The listing builds one solid part. Answer for the finished solid, in the listing's coordinates (mm). Face numbers are marked on the shaded views. A direction names the side the tool comes from. Round coordinates to 2 decimals unless told otherwise and drop trailing zeros. Order: outer loops, then holes, each group sorted by start corner. A loop starts at its lowest first (then second) coordinate and runs counter-clockwise, first axis right, second up. Notation, with made-up numbers: (60, -18) - (81, -18) arc R26 cw to (81, 0) - close; hole circle Ø11 at (-26.75, 39). An arc over 180 degrees is marked (long way). One line per item, written item: value. Start each with the question number.
1. For a pull along Z with two mould halves and no side action, classify the marked faces 3, 4 and 5 as released by +Z, released by -Z, zero draft, split by the parting line, or undercut.
2. Section D-D, the plane y = 2.65 is taken. Give the vertices of the cut face in (x, z).
3. Section C-C, the plane y = 0.4 is taken. Give the vertices of the cut face in (x, z).
4. A tool of negligible diameter and unlimited length cuts with its end or side. For the marked faces 1 and 2, from which of +Z, -Z, +X, -X, +Y, -Y can it reach the whole face along a straight path? Write none if from no direction.
5. Flat-ended cylindrical pins translate along their axes: P1, Ø2, axis at x = -3, y = 3.5, coming from the -Z side; P2, Ø4, axis at x = 0, z = 0, coming from the +Y side; P3, Ø2, axis at x = -4.5, y = 3, coming from the +Z side. Find the tip coordinate at first contact, or state that the pin passes through.
6. Straight lines are drawn through the part: line 1 (X direction, y = 0.8, z = 0); line 2 (X direction, y = 1.75, z = 0); line 3 (X direction, y = 3.5, z = -1.5). For each, find the intervals that lie inside material, in ascending order.
7. Section A-A, the plane x = -1.25 is taken. Give the vertices of the cut face in (y, z), then the cut area to 3 significant figures.
8. Section B-B, the plane z = 0 is taken. Give the vertices of the cut face in (x, y), then the cut area to 3 significant figures.
from build123d import *

# Parameters (mm, degrees)
SKETCH1_R           = 5
SKETCH1_R_2         = 2.5
BOSS_EXTRUDE1_DEPTH = 3.2
SKETCH2_R           = 5.8
SKETCH2_R_2         = 2.5
BOSS_EXTRUDE2_DEPTH = 0.8
SKETCH3_R           = 4.35508582
SKETCH3_R_2         = 3.692114727
CUT_EXTRUDE1_DEPTH  = 1
SKETCH4_R           = 4.43730614
SKETCH4_R_2         = 3.629860823
CUT_EXTRUDE2_DEPTH  = 1


with BuildPart() as part:
    # Sketch1 → Boss-Extrude1 (new body)
    with BuildSketch(Plane(origin=(0, 0, 0), x_dir=(1, 0, 0), z_dir=(0, 1, 0))):
        with Locations(Location((0, 0, 0), (0, 0, 270))):
            Circle(SKETCH1_R)
        with Locations(Location((0, 0, 0), (0, 0, 270))):
            Circle(SKETCH1_R_2, mode=Mode.SUBTRACT)
    extrude(amount=BOSS_EXTRUDE1_DEPTH)

    # Sketch2 → Boss-Extrude2 (add)
    with BuildSketch(Plane(origin=(0, 3.2, 0), x_dir=(1, 0, 0), z_dir=(0, 1, 0))):
        with Locations(Location((0, 0, 0), (0, 0, 270))):
            Circle(SKETCH2_R)
        with Locations(Location((0, 0, 0), (0, 0, 270))):
            Circle(SKETCH2_R_2, mode=Mode.SUBTRACT)
    extrude(amount=BOSS_EXTRUDE2_DEPTH)

    # Sketch3 → Cut-Extrude1 (cut)
    with BuildSketch(Plane.XZ):
        with Locations(Location((0, 0, 0), (0, 0, 270))):
            Circle(SKETCH3_R)
        with Locations(Location((0, 0, 0), (0, 0, 270))):
            Circle(SKETCH3_R_2, mode=Mode.SUBTRACT)
    extrude(amount=-CUT_EXTRUDE1_DEPTH, mode=Mode.SUBTRACT)

    # Sketch4 → Cut-Extrude2 (cut)
    with BuildSketch(Plane(origin=(0, 4, 0), x_dir=(1, 0, 0), z_dir=(0, 1, 0))):
        with Locations(Location((0, 0, 0), (0, 0, 270))):
            Circle(SKETCH4_R)
        with Locations(Location((0, 0, 0), (0, 0, 270))):
            Circle(SKETCH4_R_2, mode=Mode.SUBTRACT)
    extrude(amount=-CUT_EXTRUDE2_DEPTH, mode=Mode.SUBTRACT)


solid = part.part
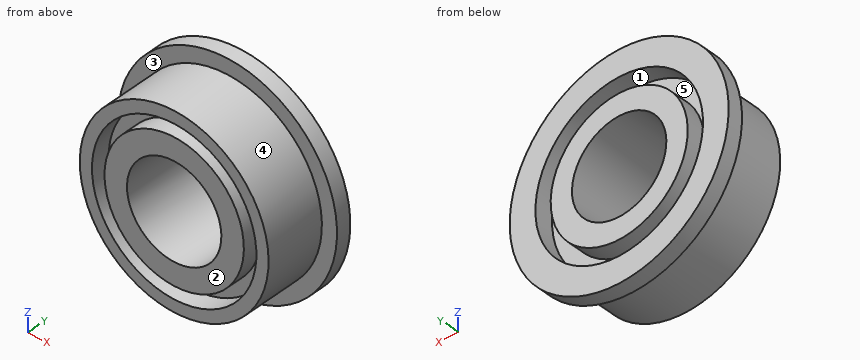
Answer list:
1. face 3: zero draft
1. face 4: split by the parting line
1. face 5: undercut
2. outline: circle Ø10 at (0, 0); hole circle Ø5 at (0, 0)
3. outline: circle Ø10 at (0, 0); circle Ø7.38 at (0, 0); hole circle Ø8.71 at (0, 0); hole circle Ø5 at (0, 0)
4. face 1: +Y
4. face 2: +Z, -Z, +X, -X, -Y
5. P1: stops at z = -5.44
5. P2: passes through
5. P3: stops at z = 4.61
6. line 1: x = -5 to -4.36, -3.69 to -2.5, 2.5 to 3.69, 4.36 to 5
6. line 2: x = -5 to -2.5, 2.5 to 5
6. line 3: x = -5.6 to -4.18, -3.31 to -2, 2 to 3.31, 4.18 to 5.6
7. outline: (0, -4.84) - (3.2, -4.84) - (3.2, -5.66) - (4, -5.66) - (4, -4.26) - (3, -4.26) - (3, -3.41) - (4, -3.41) - (4, -2.17) - (0, -2.17) - (0, -3.47) - (1, -3.47) - (1, -4.17) - (0, -4.17) - close; (0, 2.17) - (4, 2.17) - (4, 3.41) - (3, 3.41) - (3, 4.26) - (4, 4.26) - (4, 5.66) - (3.2, 5.66) - (3.2, 4.84) - (0, 4.84) - (0, 4.17) - (1, 4.17) - (1, 3.47) - (0, 3.47) - close
7. area: 19.6 mm²
8. outline: (-5.8, 3.2) - (-5, 3.2) - (-5, 0) - (-4.36, 0) - (-4.36, 1) - (-3.69, 1) - (-3.69, 0) - (-2.5, 0) - (-2.5, 4) - (-3.63, 4) - (-3.63, 3) - (-4.44, 3) - (-4.44, 4) - (-5.8, 4) - close; (2.5, 0) - (3.69, 0) - (3.69, 1) - (4.36, 1) - (4.36, 0) - (5, 0) - (5, 3.2) - (5.8, 3.2) - (5.8, 4) - (4.44, 4) - (4.44, 3) - (3.63, 3) - (3.63, 4) - (2.5, 4) - close
8. area: 18.3 mm²
